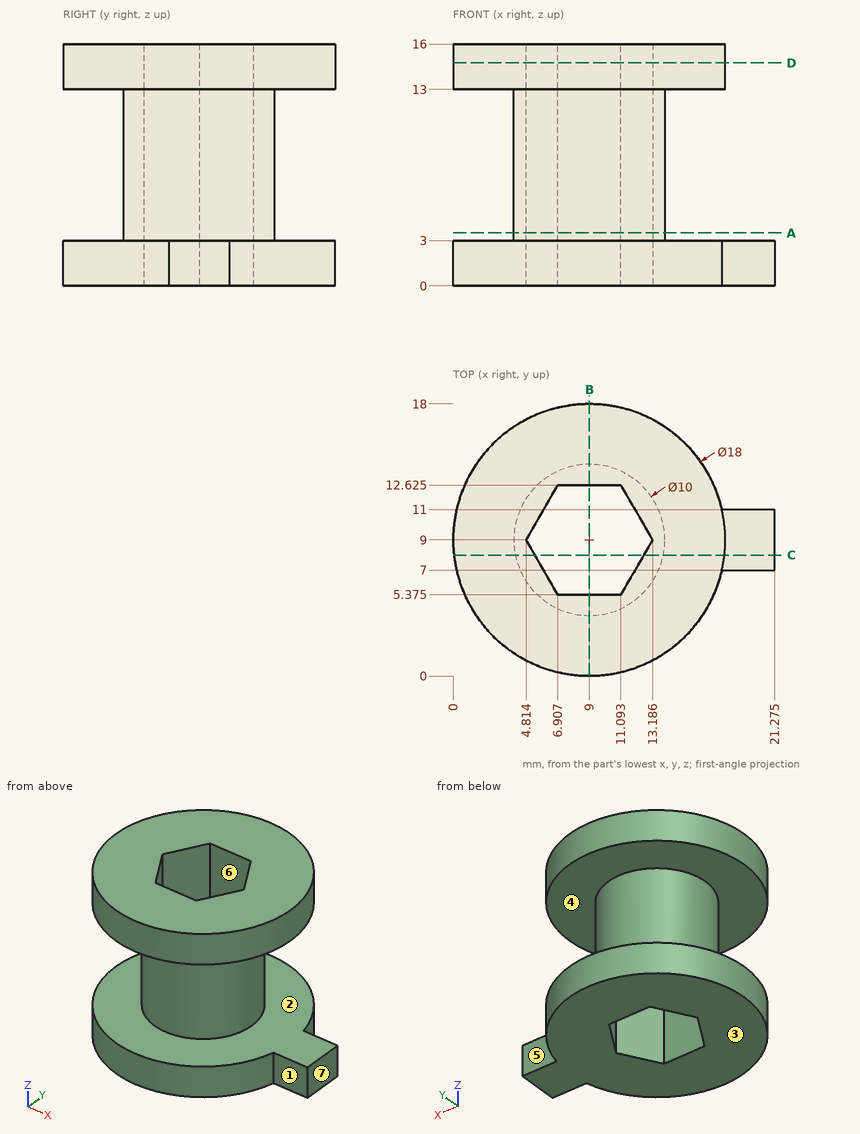
The figure shows three views and two pictorial views of one solid part (mm, origin at its lowest corner). Answer the questions. A direction names the side the tool comes from. Coordinates: 2 decimals unless noted, no trailing zeros. Loops run counter-clockwise (first coordinate to the right, second up) from the corner with the lowest first, then second, coordinate; pieces in that order, holes last. Notation, with made-up numbers: (14, 58.5) - (46, 58.5) arc R16 cw to (46, 68.5) - close; hole circle Ø6 at (58, 40.25). An arc over 180 degrees is marked (long way). Write item = value, one per line.
1) Section B-B (x = 9) is taken. Determine the outline of the cut face in (y, z) (3 decimals).
Responses:
outline = (0, 0) - (5.375, 0) - (5.375, 16) - (0, 16) - (0, 13) - (4, 13) - (4, 3) - (0, 3) - close; (12.625, 0) - (18, 0) - (18, 3) - (14, 3) - (14, 13) - (18, 13) - (18, 16) - (12.625, 16) - close
2) Determine the mould class of the marked faces 1, 2 and 3 for opening direction Z: pulls with the +Z half, pulls with the -Z half, needs draft (parallel to the pull), parting line crosses it, or undercut.
Responses:
face_1 = needs draft
face_2 = undercut
face_3 = pulls with the -Z half
3) Find the intervals of material crossed by line 1 along Z through (x, y) = (10.25, 15.5); line 2 along Y through (x, z) = (5.75, 13.75); line 3 along X through (y, z) = (6.5, 4.75), in increasing order.
Responses:
line_1 = 0 to 3, 13 to 16
line_2 = 0.61 to 7.38, 10.62 to 17.39
line_3 = 4.67 to 6.26, 11.74 to 13.33
4) Section D-D (z = 14.75) is taken. Determine the outline of the cut face in (x, y) (1 decimal), plus the area to 3 significant figures.
Responses:
outline = circle Ø18 at (9, 9); hole (4.8, 9) - (6.9, 5.4) - (11.1, 5.4) - (13.2, 9) - (11.1, 12.6) - (6.9, 12.6) - close
area = 209 mm^2
5) Each of these flat-tipped pins is pushed along its axis until it touches: P1, Ø5, axis at y = 6, z = 3.5, coming from the +X side (3 decimals); P2, Ø2, axis at x = 13, z = 12.5, coming from the +Y side; P3, Ø1.5, axis at y = 13, z = 7, coming from the +X side; P4, Ø2, axis at y = 4.5, z = 13, coming from the +X side. Where does it stop, or does it pass through?
Responses:
P1 = 21.275
P2 = 17.44
P3 = 12.8
P4 = 17.29
6) Which of the six approach directions +Z, -Z, +X, -X, +Y, -Y give full straight-line access (tool end or side, diameter ignored) to the marked faces 4, 5, 6 and 7?
Responses:
face_4 = none
face_5 = +Z, -Z, +X, +Y
face_6 = +Z, -Z
face_7 = +Z, -Z, +X, +Y, -Y
7) Section A-A (z = 3.5) is taken. Determine the outline of the cut face in (x, y) (1 decimal).
Responses:
outline = circle Ø10 at (9, 9); hole (4.8, 9) - (6.9, 5.4) - (11.1, 5.4) - (13.2, 9) - (11.1, 12.6) - (6.9, 12.6) - close
8) Section C-C (y = 8) is taken. Determine the outline of the cut face in (x, z) (1 decimal).
Responses:
outline = (0.1, 0) - (5.4, 0) - (5.4, 16) - (0.1, 16) - (0.1, 13) - (4.1, 13) - (4.1, 3) - (0.1, 3) - close; (12.6, 0) - (21.3, 0) - (21.3, 3) - (13.9, 3) - (13.9, 13) - (17.9, 13) - (17.9, 16) - (12.6, 16) - close
